```python
from build123d import *

# Parameters (mm, degrees)
SKETCH_1_R          = 26
EXTRUDE_1_DEPTH     = 3
SKETCH_2_R          = 7.5
CUT_EXTRUDE_1_DEPTH = 37.891733491
EXTRUDE_START       = 5
SKETCH_3_R          = 8.5
SKETCH_3_R_2        = 7.5
EXTRUDE_3_DEPTH     = 5
SKETCH_4_R          = 1.35
CUT_EXTRUDE_2_DEPTH = 38.107950631
SKETCH_5_R          = 2
CUT_EXTRUDE_3_DEPTH = 1


with BuildPart() as part:
    # Эскиз1 → Бобышка-Вытянуть1 (new body)
    with BuildSketch(Plane.XY):
        Circle(SKETCH_1_R)
    extrude(amount=EXTRUDE_1_DEPTH)

    # Эскиз2 → Вырез-Вытянуть1 (cut, through all)
    with BuildSketch(Plane.XY.offset(3)):
        Circle(SKETCH_2_R)
    extrude(amount=-CUT_EXTRUDE_1_DEPTH, mode=Mode.SUBTRACT)

    # Эскиз3 → Бобышка-Вытянуть3 (add)
    with BuildSketch(Plane.XY.offset(3).offset(EXTRUDE_START)):
        Circle(SKETCH_3_R)
        Circle(SKETCH_3_R_2, mode=Mode.SUBTRACT)
    extrude(amount=-EXTRUDE_3_DEPTH)

    # Эскиз4 → Вырез-Вытянуть2 (cut, through all)
    with BuildSketch(Plane.XY.offset(3)):
        with Locations((-15.556349186, 15.556349186)):
            Circle(SKETCH_4_R)
        with Locations((15.556349186, 15.556349186)):
            Circle(SKETCH_4_R)
        with Locations((15.556349186, -15.556349186)):
            Circle(SKETCH_4_R)
        with Locations((-15.556349186, -15.556349186)):
            Circle(SKETCH_4_R)
    extrude(amount=-CUT_EXTRUDE_2_DEPTH, mode=Mode.SUBTRACT)

    # Эскиз5 → Вырез-Вытянуть3 (cut)
    with BuildSketch(Plane.XY.offset(3)):
        with Locations((-15.556349186, 15.556349186)):
            Circle(SKETCH_5_R)
        with Locations((15.556349186, 15.556349186)):
            Circle(SKETCH_5_R)
        with Locations((15.556349186, -15.556349186)):
            Circle(SKETCH_5_R)
        with Locations((-15.556349186, -15.556349186)):
            Circle(SKETCH_5_R)
    extrude(amount=-CUT_EXTRUDE_3_DEPTH, mode=Mode.SUBTRACT)


solid = part.part
```
Geometry: final body of the model. Coordinates: model frame, mm. A direction names the side the tool comes from. Coordinates: 2 decimals unless noted, no trailing zeros. Write each loop counter-clockwise with the first axis right and the second up, starting at its lowest first coordinate (ties: lowest second). Pieces come first, ordered by that corner, then holes. Notation, with made-up numbers: M 25,-26.5 L 52,-26.5 A4 cw 52,-22.5 Z; hole C 51,79.25 d11. An arc over 180 degrees is marked long. Use CSV: the item, a comma, the result in double quotes. Start each with the question number.
1. Mould query, pull axis Y, two halves, no side actions, for faces 1 (the face through (-20.633, -15.821, 1.479)), 2 (the face through (-15, -17, 2)), 3 (the face through (-6.14, 6.14, 3)). Classes: pulls with the +Y half, pulls with the -Y half, needs draft (parallel to the pull), parting line crosses it, or undercut.
2. Cut plane D-D on y = -12.5. Return the cut outline in (x, z), plus the area to 3 significant figures.
3. Reachability of faces 4 (the face through (0, -8, 8)), 5 (the face through (-17.554, 15.644, 2.507)) from +Z, -Z, +X, -X, +Y, -Y: full face, straight path, thin tool, end or side. Return the list, or none.
4. Ray query, probe 1 along X at (y, z) = (-15, 2.75); probe 2 along X at (y, z) = (1, 1.5); probe 3 along Y at (x, z) = (6, 7.25). Return the intervals inside material, ascending.
5. Cut plane C-C on z = 3.75. Return the cut outline in (x, y), plus the area to 3 significant figures.
6. First-contact query: P1, Ø2.5, axis at x = 15.56, y = 15.56, coming from the -Z side; P2, Ø2, axis at x = -20.5, z = 3.5, coming from the +Y side; P3, Ø2, axis at x = -15, y = -16, coming from the +Z side; P4, Ø3, axis at x = -11.5, y = -2.5, coming from the +Z side. Flat tips, straight axial feed; report the tip coordinate or a pass-through.
7. Cut plane A-A on y = 0. Return the cut outline in (x, z).
Entries:
1,face 1,"parting line crosses it"
1,face 2,"undercut"
1,face 3,"needs draft"
2,outline,"M -22.8,0 L 22.8,0 L 22.8,3 L -22.8,3 Z"
2,area,"137 mm²"
3,face 4,"+Z, +X, -X, +Y, -Y"
3,face 5,"+Z"
4,probe 1,"-21.24 to -17.48, -13.64 to 13.64, 17.48 to 21.24"
4,probe 2,"-25.98 to -7.43, 7.43 to 25.98"
4,probe 3,"-6.02 to -4.5, 4.5 to 6.02"
5,outline,"C 0,0 d17; hole C 0,0 d15"
5,area,"50.3 mm²"
6,P1,"through"
6,P2,"y = 17.04"
6,P3,"z = 2"
6,P4,"z = 3"
7,outline,"M -26,0 L -7.5,0 L -7.5,8 L -8.5,8 L -8.5,3 L -26,3 Z; M 7.5,0 L 26,0 L 26,3 L 8.5,3 L 8.5,8 L 7.5,8 Z"
